Read the model definition and answer for the solid it produces. Units are mm, in the model's axes. A direction names the side the tool comes from. Coordinates: 2 decimals unless noted, no trailing zeros. Write each loop counter-clockwise with the first axis right and the second up, starting at its lowest first coordinate (ties: lowest second). Pieces come first, ordered by that corner, then holes. Notation, with made-up numbers: (55.5, 64.25) -> (69.5, 64.25) arc R27 ccw to (69.5, 87.25) -> close; hole circle Ø2 at (63.25, 41.25). An arc over 180 degrees is marked (long way). Return JSON: item names as keys, results as strings.
Autodesk Inventor part; units mm, degrees
ref_plane "YZ Plane" through (0, 0, 0) normal (1, 0, 0) x (0, 1, 0)
ref_plane "XZ Plane" through (0, 0, 0) normal (0, 1, 0) x (-1, 0, 0)
ref_plane "XY Plane" through (0, 0, 0) normal (0, 0, 1) x (1, 0, 0)
sketch "Sketch1" plane through (0, 0, 0) normal (0, 0, 1) x (1, 0, 0)
  line L0 (0, 0) -> (2400, 0)
  line L1 (2400, 0) -> (2400, -800)
  line L2 (2400, -800) -> (0, -800)
  line L3 (0, -800) -> (0, 0)
  line L4 (0, 0) -> (575, 0)
  line L5 (575, 0) -> (575, -125)
  line L6 (0, 0) -> (1775, 0)
  line L7 (1775, 0) -> (1775, -125)
  circle A0 centre (575, -125) radius 100
  circle A1 centre (1775, -125) radius 100
  dimension "d0" = 2400
  dimension "d1" = 800
  dimension "d2" = 575
  dimension "d3" = 125
  dimension "d4" = 1775
  dimension "d5" = 200
extrude "Extrusion1" add sketch "Sketch1" along normal blind 35 contours A1 | A0
extrude "Extrusion2" add sketch "Sketch1" against normal blind 100
sketch "Sketch2" plane through (575, -125, 35) normal (0, 0, 1) x (1, 0, 0)
  point P0 (-575, 125)
extrude "Extrusion3" add sketch "Sketch1" against normal blind 100 contours A0
extrude "Extrusion4" add sketch "Sketch1" against normal blind 100 contours A1
sketch "Sketch3" plane through (0, 0, -100) normal (0, 0, -1) x (-1, 0, 0)
  point P0 (0, 0)
sketch "Sketch4" plane through (0, 0, -100) normal (0, 0, -1) x (-1, 0, 0)
  line L0 (0, 0) -> (-2400, 0)
  line L1 (0, 0) -> (0, -40)
  line L2 (0, -800) -> (0, 0)
  line L3 (0, -40) -> (-40, -40)
  line L4 (-40, -40) -> (-110, -40)
  line L5 (-110, -40) -> (-110, -110)
  line L6 (-110, -110) -> (-40, -110)
  line L7 (-40, -110) -> (-40, -40)
  line L8 (-2400, -800) -> (0, -800)
  line L9 (0, -800) -> (-40, -800)
  line L10 (0, -760) -> (0, -800)
  line L11 (-40, -760) -> (-110, -760)
  line L12 (-110, -760) -> (-110, -690)
  line L13 (-110, -690) -> (-40, -690)
  line L14 (-40, -690) -> (-40, -760)
  line L15 (-2400, 0) -> (-2400, -800)
  line L16 (-2400, 0) -> (-2400, -40)
  line L17 (-2400, -40) -> (-2360, -40)
  line L18 (-2400, -800) -> (-2400, -760)
  line L19 (-2400, -760) -> (-2360, -760)
  line L20 (-2360, -40) -> (-2290, -40)
  line L21 (-2290, -40) -> (-2290, -110)
  line L22 (-2290, -110) -> (-2360, -110)
  line L23 (-2360, -110) -> (-2360, -40)
  line L24 (-2360, -760) -> (-2290, -760)
  line L25 (-2290, -760) -> (-2290, -690)
  line L26 (-2290, -690) -> (-2360, -690)
  line L27 (-2360, -690) -> (-2360, -760)
  dimension "d14" = 40
  dimension "d15" = 40
  dimension "d16" = 70
  dimension "d17" = 70
  dimension "d18" = 40
  dimension "d19" = 40
  dimension "d20" = 70
  dimension "d21" = 70
  dimension "d22" = 40
  dimension "d23" = 40
  dimension "d24" = 70
  dimension "d25" = 70
  dimension "d26" = 70
  dimension "d27" = 70
extrude "Extrusion5" add sketch "Sketch4" along normal blind 800 contours L20 L21 L22 L23 | L27 L26 L25 L24 | L7 L6 L5 L4 | L11 L12 L13 L14
properties part number "Master-workspace"
1. For a pull along Y with two mould halves and no side action, classify faces 1 (the face through (2325, -40, -494)), 2 (the face through (2360, -725, -494)), 3 (the face through (75, -110, -494)) as +Y half, -Y half, draft (parallel to the pull), parting line (faces both ways), or undercut.
Taken from the geometry:
{"face 1": "+Y half", "face 2": "draft", "face 3": "undercut"}
2. Flat-ended cylindrical pins translate along their axes: pin 1 Ø5 at (x, y) = (571.5, -710.5) entering from -Z; pin 2 Ø21 at (x, z) = (88.5, -302) entering from +Y; pin 3 Ø21 at (y, z) = (-80.5, -580.5) entering from +X. Find the tip coordinate at first contact, or state that the pin passes through.
Taken from the geometry:
{"pin 1": "stops at z = -100", "pin 2": "stops at y = -40", "pin 3": "stops at x = 2360"}
3. The part is cut by section B-B (x = 1775). Determine the outline of the cut face in (y, z), then the cut area to 3 significant figures.
Taken from the geometry:
{"outline": "(-800, -100) -> (0, -100) -> (0, 0) -> (-25, 0) -> (-25, 35) -> (-225, 35) -> (-225, 0) -> (-800, 0) -> close", "area": "87,000 mm2"}
4. The part is cut by section A-A (z = -486). Determine the outline of the cut face in (x, y).
Taken from the geometry:
{"outline": "(40, -760) -> (110, -760) -> (110, -690) -> (40, -690) -> close; (40, -110) -> (110, -110) -> (110, -40) -> (40, -40) -> close; (2290, -760) -> (2360, -760) -> (2360, -690) -> (2290, -690) -> close; (2290, -110) -> (2360, -110) -> (2360, -40) -> (2290, -40) -> close"}
5. The part is cut by section D-D (x = 1041.5). Determine the outline of the cut face in (y, z), then the cut area to 3 significant figures.
Taken from the geometry:
{"outline": "(-800, -100) -> (0, -100) -> (0, 0) -> (-800, 0) -> close", "area": "80,000 mm2"}
6. The part is cut by section C-C (y = -364.5). Determine the outline of the cut face in (x, z).
Taken from the geometry:
{"outline": "(0, -100) -> (2400, -100) -> (2400, 0) -> (0, 0) -> close"}
7. Consider L1, parallel to Z at x = 1470, y = -579; L2, parallel to X at y = -81.5, z = -657; L3, parallel to Z at x = 1726, y = -212. Determine where each line is inside the solid, lowest interval first.
Taken from the geometry:
{"L1": "z = -100 to 0", "L2": "x = 40 to 110, 2290 to 2360", "L3": "z = -100 to 35"}
8. A tool of negligible diameter and unlimited length cuts with its end or side. For faces 4 (the face through (2290, -725, -494)), 5 (the face through (75, -690, -494)), 6 (the face through (2325, -760, -494)), 7 (the face through (1870.38, -155.04, 17.26)), from which of +Z, -Z, +X, -X, +Y, -Y can it reach the whole face along a straight path? Write none if from no direction.
Taken from the geometry:
{"face 4": "-Z, +Y, -Y", "face 5": "-Z, +X, -X", "face 6": "-Z, +X, -X, -Y", "face 7": "+Z"}
